Work out the finished part from the listing and answer in its coordinate system (mm). Face numbers are marked on the shaded views. A direction names the side the tool comes from. Round coordinates to 2 decimals unless told otherwise and drop trailing zeros. Order: outer loops, then holes, each group sorted by start corner. A loop starts at its lowest first (then second) coordinate and runs counter-clockwise, first axis right, second up. Notation, with made-up numbers: (-2.75, -24.5) -> (23.25, -24.5) arc R20 ccw to (23.25, -4.5) -> close; hole circle Ø4 at (-17, 41). An arc over 180 degrees is marked (long way). Use a Markdown table: item, result. Add a question column.
Item 1: For a pull along X with two mould halves and no side action, classify the marked faces 3, 4, 5 and 6 as +X half, -X half, draft (parallel to the pull), parting line (faces both ways), or undercut.
Item 2: A cutting plane is placed at D-D, the plane x = -49. Determine the outline of the cut face in (y, z), plus the area to 3 significant figures.
Item 3: A cutting plane is placed at B-B, the plane x = 6.35. Determine the outline of the cut face in (y, z), plus the area to 3 significant figures.
Item 4: Find the intervals of material crossed by L1, parallel to X at y = 1.95, z = 3.81; L2, parallel to Z at x = -6.35, y = 0.95; L3, parallel to Y at x = -21, z = -1.5, in increasing order. Write a range as [from, to].
Item 5: A tool of negligible diameter and unlimited length cuts with its end or side. For the marked faces 1 and 2, from which of +Z, -Z, +X, -X, +Y, -Y can it reach the whole face along a straight path? Write none if from no direction.
Item 6: A cutting plane is placed at A-A, the plane y = -42.5. Determine the outline of the cut face in (x, z), plus the area to 3 significant figures.
from build123d import *

# Parameters (mm, degrees)
SKETCH1_R           = 1.5875
SKETCH1_W           = 7.62
SKETCH1_H           = 5.08
BOSS_EXTRUDE1_DEPTH = 2.54
SKETCH2_W           = 2.54
SKETCH2_H           = 12.7
BOSS_EXTRUDE2_DEPTH = 50.8
SKETCH3_W           = 127
SKETCH3_H           = 12.7
BOSS_EXTRUDE3_DEPTH = 2.54
FILLET1_R           = 2.54
FILLET2_R           = 3.175


with BuildPart() as part:
    # Sketch1 → Boss-Extrude1 (new body)
    with BuildSketch(Plane(origin=(0, 0, 0), x_dir=(1, 0, 0), z_dir=(0, 1, 0))):
        Polygon((-63.5, 6.35), (-12.7, 6.35), (12.7, 6.35), (63.5, 6.35), (63.5, -6.35), (12.7, -6.35), (-12.7, -6.35), (-63.5, -6.35), align=None)
        with Locations((-6.35, 3.81)):
            Circle(SKETCH1_R, mode=Mode.SUBTRACT)
        with Locations((6.35, 3.81)):
            Circle(SKETCH1_R, mode=Mode.SUBTRACT)
        with Locations((6.35, -3.81)):
            Circle(SKETCH1_R, mode=Mode.SUBTRACT)
        with Locations((-6.35, -3.81)):
            Circle(SKETCH1_R, mode=Mode.SUBTRACT)
        Rectangle(SKETCH1_W, SKETCH1_H, mode=Mode.SUBTRACT)
    extrude(amount=BOSS_EXTRUDE1_DEPTH)

    # Sketch2 → Boss-Extrude2 (add)
    with BuildSketch(Plane.XZ):
        with Locations((-62.23, 0)):
            Rectangle(SKETCH2_W, SKETCH2_H)
        with Locations((62.23, 0)):
            Rectangle(SKETCH2_W, SKETCH2_H)
    extrude(amount=BOSS_EXTRUDE2_DEPTH)

    # Sketch3 → Boss-Extrude3 (add)
    with BuildSketch(Plane.XZ.offset(50.8)):
        Rectangle(SKETCH3_W, SKETCH3_H)
    extrude(amount=-BOSS_EXTRUDE3_DEPTH)

    # Fillet1
    fillet1_edges = [part.edges().sort_by_distance(p)[0] for p in [
        (-60.96, -48.26, 0),
        (60.96, -48.26, 0),
    ]]
    fillet(fillet1_edges, radius=FILLET1_R)

    # Fillet2
    fillet2_edges = [part.edges().sort_by_distance(p)[0] for p in [
        (-60.96, 0, 0),
        (60.96, 0, 0),
    ]]
    fillet(fillet2_edges, radius=FILLET2_R)


solid = part.part
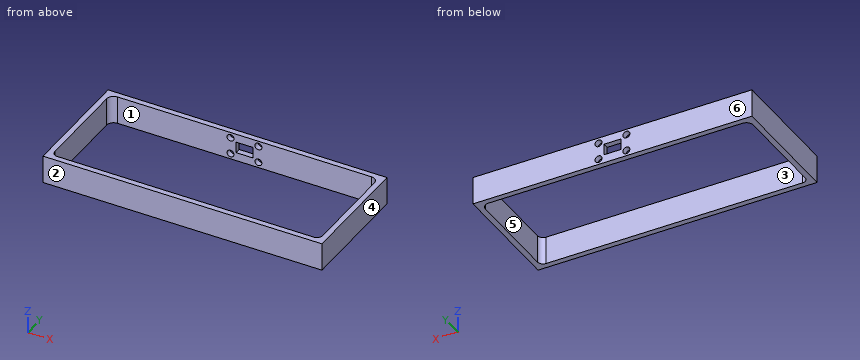
Reported:
| question | item | result |
|---|---|---|
| 1 | face 3 | undercut |
| 1 | face 4 | +X half |
| 1 | face 5 | undercut |
| 1 | face 6 | draft |
| 2 | outline | (-50.8, -6.35) -> (-48.26, -6.35) -> (-48.26, 6.35) -> (-50.8, 6.35) -> close; (0, -6.35) -> (2.54, -6.35) -> (2.54, 6.35) -> (0, 6.35) -> close |
| 2 | area | 64.5 mm² |
| 3 | outline | (-50.8, -6.35) -> (-48.26, -6.35) -> (-48.26, 6.35) -> (-50.8, 6.35) -> close; (0, -6.35) -> (2.54, -6.35) -> (2.54, -5.4) -> (0, -5.4) -> close; (0, -2.22) -> (2.54, -2.22) -> (2.54, 2.22) -> (0, 2.22) -> close; (0, 5.4) -> (2.54, 5.4) -> (2.54, 6.35) -> (0, 6.35) -> close |
| 3 | area | 48.4 mm² |
| 4 | L1 | [-63.5, -7.94], [-4.76, 4.76], [7.94, 63.5] |
| 4 | L2 | [-6.35, -5.4], [-2.22, 2.22], [5.4, 6.35] |
| 4 | L3 | [-50.8, -48.26], [0, 2.54] |
| 5 | face 1 | +Z, -Z |
| 5 | face 2 | +Z, -Z, +X, -X, -Y |
| 6 | outline | (-63.5, -6.35) -> (-60.96, -6.35) -> (-60.96, 6.35) -> (-63.5, 6.35) -> close; (60.96, -6.35) -> (63.5, -6.35) -> (63.5, 6.35) -> (60.96, 6.35) -> close |
| 6 | area | 64.5 mm² |
